Autodesk Inventor part; units mm, degrees
ref_plane "YZ Plane" through (0, 0, 0) normal (1, 0, 0) x (0, 1, 0)
ref_plane "XZ Plane" through (0, 0, 0) normal (0, 1, 0) x (-1, 0, 0)
ref_plane "XY Plane" through (0, 0, 0) normal (0, 0, 1) x (1, 0, 0)
sketch "Sketch1" plane through (0, 0, 0) normal (0, 1, 0) x (-1, 0, 0)
  line L0 (144.8249, 258.4464) -> (-105.1751, 258.4464)
  line L1 (-105.1751, 258.4464) -> (-105.1751, -361.5536)
  line L2 (-105.1751, -361.5536) -> (144.8249, -361.5536)
  line L3 (144.8249, -361.5536) -> (144.8249, 258.4464)
  point P0 (0, 0)
  dimension "d0" = 620
  dimension "d1" = 250
extrude "Extrusion1" add sketch "Sketch1" along normal blind 200
sketch "Sketch2" plane through (0, 200, 0) normal (0, 1, 0) x (1, 0, 0)
  line L0 (89.2369, -235.4618) -> (-130.7631, -235.4618)
  line L1 (-130.7631, -235.4618) -> (-130.7631, 114.5382)
  line L2 (-130.7631, 114.5382) -> (89.2369, 114.5382)
  line L3 (89.2369, 114.5382) -> (89.2369, -235.4618)
  point P0 (0, 0)
  dimension "d4" = 220
  dimension "d5" = 350
extrude "Extrusion2" cut sketch "Sketch2" against normal blind 185
sketch "Sketch3" plane through (0, 200, 0) normal (0, 1, 0) x (1, 0, 0)
  line L0 (-126.25, 127.5) -> (83.75, 127.5)
  line L1 (83.75, 127.5) -> (83.75, 322.5)
  line L2 (83.75, 322.5) -> (-126.25, 322.5)
  line L3 (-126.25, 322.5) -> (-126.25, 127.5)
  point P0 (0, 0)
  dimension "d8" = 210
  dimension "d9" = 195
extrude "Extrusion3" cut sketch "Sketch3" against normal blind 185
properties part number "collector"
The listing builds one solid part. Answer for the finished solid, in the listing's coordinates (mm). A direction names the side the tool comes from. Give positions to 0.01 mm unless a question says otherwise; leave off trailing zeros. Loops run counter-clockwise (first coordinate to the right, second up) from the corner with the lowest first, then second, coordinate; pieces in that order, holes last. Notation, with made-up numbers: M -12.75,1.5 L 39.25,1.5 A5 ccw 39.25,6.5 Z; hole C 15,40 d4. An arc over 180 degrees is marked long. One line per item, written item: value.
Q1. A cutting plane is placed at A-A on y = 41.5. Determine the outline of the cut face in (x, z).
Working result:
outline: M -144.82,-361.55 L 105.18,-361.55 L 105.18,258.45 L -144.82,258.45 Z; hole M -130.76,-114.54 L 89.24,-114.54 L 89.24,235.46 L -130.76,235.46 Z; hole M -126.25,-322.5 L 83.75,-322.5 L 83.75,-127.5 L -126.25,-127.5 Z
Q2. A cutting plane is placed at B-B on x = -105.5. Determine the outline of the cut face in (y, z).
Working result:
outline: M 0,-361.55 L 200,-361.55 L 200,-322.5 L 15,-322.5 L 15,-127.5 L 200,-127.5 L 200,-114.54 L 15,-114.54 L 15,235.46 L 200,235.46 L 200,258.45 L 0,258.45 Z
Q3. Find the intervals of material crossed by line 1 (Z direction, x = 16.5, y = 174); line 2 (X direction, y = 131, z = -191.5); line 3 (X direction, y = 76, z = -36.5), in increasing order. Write a range as from..to.
Working result:
line 1: z = -361.55..-322.5, -127.5..-114.54, 235.46..258.45
line 2: x = -144.82..-126.25, 83.75..105.18
line 3: x = -144.82..-130.76, 89.24..105.18
Q4. Determine the mould class of faces 3 (the face through (-23, 15, -226)), 4 (the face through (-144.825, 99, -56)), 5 (the face through (-18, 99, -361.554)) for opening direction X: +X half, -X half, draft (parallel to the pull), parting line (faces both ways), or undercut.
Working result:
face 3: undercut
face 4: -X half
face 5: draft
Q5. A cutting plane is placed at C-C on z = -27. Determine the outline of the cut face in (x, y).
Working result:
outline: M -144.82,0 L 105.18,0 L 105.18,200 L 89.24,200 L 89.24,15 L -130.76,15 L -130.76,200 L -144.82,200 Z
Q6. A cutting plane is placed at D-D on z = -303.5. Determine the outline of the cut face in (x, y).
Working result:
outline: M -144.82,0 L 105.18,0 L 105.18,200 L 83.75,200 L 83.75,15 L -126.25,15 L -126.25,200 L -144.82,200 Z
Q7. Flat-ended cylindrical pins translate along their axes: P1, Ø5, axis at x = 57, z = -160.5, coming from the +Y side; P2, Ø1.5, axis at x = -51, z = -243, coming from the -Y side. Find the tip coordinate at first contact, or state that the pin passes through.
Working result:
P1: stops at y = 15
P2: stops at y = 0
Q8. For faces 1 (the face through (-126.25, 109, -226)), 2 (the face through (105.175, 99, -47)), determine the directions among +Z, -Z, +X, -X, +Y, -Y from which every point of the face is accessible in a straight line to the end or side of a thin tool.
Working result:
face 1: +Y
face 2: +Z, -Z, +X, +Y, -Y
